```python
from build123d import *

# Parameters (mm, degrees)
F0_R     = 24.765
F1_DEPTH = 7.62
F2_R     = 28.575
F3_DEPTH = 15.875
F4_SIZE2 = 12.7
F4_SIZE  = 12.7
F5_R     = 10.31875
F6_DEPTH = 23.496
F7_SIZE  = 0.79375


with BuildPart() as f1:
    # F0 (on Top) → F1 (new body)
    with BuildSketch(Plane.XY):
        Circle(F0_R)
    extrude(amount=F1_DEPTH)

    # F2 (on face) → F3 (join)
    with BuildSketch(Plane.XY.offset(7.62)):
        Circle(F2_R)
    extrude(amount=F3_DEPTH)

    # F4
    f4_edges = [f1.edges().sort_by_distance(p)[0] for p in [
        (-28.575, 0, 23.495),
    ]]
    chamfer(f4_edges, length=F4_SIZE, length2=F4_SIZE2)

    # F5 (on face) → F6 (cut, through all)
    with BuildSketch(Plane.XY.offset(23.495)):
        Circle(F5_R)
    extrude(amount=-F6_DEPTH, mode=Mode.SUBTRACT)

    # F7
    f7_edges = [f1.edges().sort_by_distance(p)[0] for p in [
        (-24.765, 0, 0),
    ]]
    chamfer(f7_edges, length=F7_SIZE)


solid = f1.part
```
Can you work these out from the model? Positions are in its coordinate system, mm. Give positions to 0.01 mm unless a question says otherwise; leave off trailing zeros. Loops run counter-clockwise (first coordinate to the right, second up) from the corner with the lowest first, then second, coordinate; pieces in that order, holes last. Notation, with made-up numbers: M 48.25,-29 L 70.25,-29 A14 cw 70.25,-15 Z; hole C -14.5,31.5 d2. An arc over 180 degrees is marked long. Use CSV: the item, a comma, the result in double quotes. Start each with the question number.
1. If I drill on L1, parallel to Y at x = 0, z = 9 (3 decimals); L2, parallel to X at y = 8.5, z = 4.75; L3, parallel to Y at x = 0, z = 16.5, over which ranges is the centre line in solid material (lowest first)?
2. Imagine slicing it at C-C, the plane z = 4. Write out the boundary of the cut face in (x, y) (1 decimal), plus the area to 3 significant figures.
3. For P1, Ø2, axis at x = -18, z = 11.5, coming from the +Y side; P2, Ø8, axis at x = -21.5, y = -9, coming from the +Z side; P3, Ø4, axis at y = -9, z = 7, coming from the +X side; P4, Ø1, axis at x = 20.5, z = 21, coming from the +Y side, each with a flat end and sliding along its axis, tell me the tip position at first contact or that it passes through.
4. If we mould it in two halves opening along X, with no side actions, what happens to faces 1 (the face through (-2.237, -10.073, 11.912)), 2 (the face through (23.62, 7.44, 4.16)), 3 (the face through (-8.6, 23.4, 7.62))? For each: released by +X, released by -X, zero draft, split by the parting line, or undercut.
5. Imagine slicing it at A-A, the plane y = 0. Write out the boundary of the cut face in (x, z) (3 decimals), plus the area to 3 significant figures.
Response values:
1,L1,"-28.575 to -10.319, 10.319 to 28.575"
1,L2,"-23.26 to -5.85, 5.85 to 23.26"
1,L3,"-22.87 to -10.32, 10.32 to 22.87"
2,outline,"C 0,0 d49.5; hole C 0,0 d20.6"
2,area,"1,590 mm^2"
3,P1,"y = 22.75"
3,P2,"z = 20.06"
3,P3,"x = 27.68"
3,P4,"through"
4,face 1,"undercut"
4,face 2,"split by the parting line"
4,face 3,"zero draft"
5,outline,"M -28.575,7.62 L -24.765,7.62 L -24.765,0.794 L -23.971,0 L -10.319,0 L -10.319,23.495 L -15.875,23.495 L -28.575,10.795 Z; M 10.319,0 L 23.971,0 L 24.765,0.794 L 24.765,7.62 L 28.575,7.62 L 28.575,10.795 L 15.875,23.495 L 10.319,23.495 Z"
5,area,"638 mm^2"
